from build123d import *

# Parameters (mm, degrees)
SKETCH3_R           = 20
BOSS_EXTRUDE1_DEPTH = 8
SKETCH4_R           = 3.75
CUT_EXTRUDE1_DEPTH  = 8
CIRPATTERN1_COUNT   = 6
CHAMFER1_SIZE       = 0.5


with BuildPart() as part:
    # Sketch3 → Boss-Extrude1 (new body)
    with BuildSketch(Plane.XY):
        Circle(SKETCH3_R)
    extrude(amount=BOSS_EXTRUDE1_DEPTH)

    # Sketch4 → Cut-Extrude1 (cut)
    with BuildSketch(Plane.XY.offset(8)):
        with Locations((0, 10)):
            Circle(SKETCH4_R)
    cut_extrude1 = extrude(amount=-CUT_EXTRUDE1_DEPTH, mode=Mode.SUBTRACT)

    # CirPattern1: Cut-Extrude1 ×6 about axis
    cirpattern1_axis = Axis((0, 0, 0), (0, 0, 1))
    for i in range(1, CIRPATTERN1_COUNT):
        add(cut_extrude1.rotate(cirpattern1_axis, i * 360 / CIRPATTERN1_COUNT), mode=Mode.SUBTRACT)

    # Chamfer1
    chamfer1_edges = [part.edges().sort_by_distance(p)[0] for p in [
        (-10.535254038, 1.752404736, 0),
        (-10.535254038, 1.752404736, 8),
        (-6.785254038, -8.247595264, 0),
        (-6.785254038, -8.247595264, 8),
        (3.75, -10, 0),
        (-20, 0, 0),
        (3.75, -10, 8),
        (10.535254038, -1.752404736, 0),
        (10.535254038, -1.752404736, 8),
        (6.785254038, 8.247595264, 0),
        (6.785254038, 8.247595264, 8),
        (-20, 0, 8),
        (-3.75, 10, 0),
        (-3.75, 10, 8),
    ]]
    chamfer(chamfer1_edges, length=CHAMFER1_SIZE)


solid = part.part
Input: part model. Units: mm. Frame: model coordinates. Give positions to 0.01 mm unless a question says otherwise; leave off trailing zeros. Order: outer loops, then holes, each group sorted by start corner. A loop starts at its lowest first (then second) coordinate and runs counter-clockwise, first axis right, second up. Notation, with made-up numbers: (89.5, 23) - (96.5, 23) arc R21 ccw to (96.5, 49) - close; hole circle Ø2 at (39, 53). An arc over 180 degrees is marked (long way). Write each question's results on one line, items separated by ' | '.
Item 1: Section C-C (y = -7.5). Give the number of separate pieces and of enclosed holes in the cut face, and give its area (3 significant figures).
A:
separate pieces: 4 | enclosed holes: 0 | area: 160 mm^2
Item 2: Contact query for flat-ended pins moving along their axis: pin 1 Ø4.5 at (x, y) = (0, 10) entering from -Z; pin 2 Ø1.5 at (x, z) = (-8.5, 5) entering from -Y; pin 3 Ø2 at (y, z) = (2.5, 4.5) entering from -X; pin 4 Ø3 at (x, z) = (14.5, 6) entering from -Y. Output: stop coordinate, or through.
A:
pin 1: passes through | pin 2: stops at y = -18.44 | pin 3: stops at x = -19.94 | pin 4: stops at y = -15.2
Item 3: Section B-B (z = 2.25). Return loops of the section in (x, y).
A:
outline: circle Ø40 at (0, 0); hole circle Ø7.5 at (-8.66, -5); hole circle Ø7.5 at (-8.66, 5); hole circle Ø7.5 at (0, -10); hole circle Ø7.5 at (0, 10); hole circle Ø7.5 at (8.66, -5); hole circle Ø7.5 at (8.66, 5)
Item 4: Material intervals for line 1 along Y through (x, z) = (0, 5.75); line 2 along Y through (x, z) = (-11.5, 1.5); line 3 along X through (y, z) = (-4.5, 3.5), sorted ascending.
A:
line 1: y = -20 to -13.75, -6.25 to 6.25, 13.75 to 20 | line 2: y = -16.36 to -7.45, -2.55 to 2.55, 7.45 to 16.36 | line 3: x = -19.49 to -12.38, -4.94 to 4.94, 12.38 to 19.49
Item 5: Section A-A (x = 0). Return loops of the section in (y, z).
A:
outline: (-20, 0.5) - (-19.5, 0) - (-14.25, 0) - (-13.75, 0.5) - (-13.75, 7.5) - (-14.25, 8) - (-19.5, 8) - (-20, 7.5) - close; (-6.25, 0.5) - (-5.75, 0) - (5.75, 0) - (6.25, 0.5) - (6.25, 7.5) - (5.75, 8) - (-5.75, 8) - (-6.25, 7.5) - close; (13.75, 0.5) - (14.25, 0) - (19.5, 0) - (20, 0.5) - (20, 7.5) - (19.5, 8) - (14.25, 8) - (13.75, 7.5) - close
